```python
from build123d import *

# Parameters (mm, degrees)
F0_W     = 190
F0_H     = 20
F1_DEPTH = 4
F2_R     = 6
F3_DEPTH = 4.001
F4_R     = 9.99999


# Not quite as in the source:
# - a fillet or chamfer is up to 0.001 mm smaller than in the source, because OpenCascade refuses the exact size


with BuildPart() as f1:
    # F0 (on Top) → F1 (new body)
    with BuildSketch(Plane.XY):
        Rectangle(F0_W, F0_H)
    extrude(amount=F1_DEPTH)

    # F2 (on face) → F3 (cut, through all)
    with BuildSketch(Plane.XY.offset(4)):
        with Locations((-85, 0)):
            Circle(F2_R)
        with Locations((27, 0)):
            Circle(F2_R)
    extrude(amount=-F3_DEPTH, mode=Mode.SUBTRACT)

    # F4 (radius 10 in the source; OpenCascade refuses exactly that, so slightly less here)
    f4_edges = [f1.edges().sort_by_distance(p)[0] for p in [
        (-95, -10, 2),
        (-95, 10, 2),
        (95, 10, 2),
        (95, -10, 2),
    ]]
    fillet(f4_edges, radius=F4_R)


solid = f1.part
```
Part model, mm, in its own coordinate system. Round coordinates to 2 decimals unless told otherwise and drop trailing zeros. Loops run counter-clockwise (first coordinate to the right, second up) from the corner with the lowest first, then second, coordinate; pieces in that order, holes last. Notation, with made-up numbers: (89.5, 24.25) -> (136.5, 24.25) arc R20 cw to (136.5, 41.25) -> close; hole circle Ø3 at (12.5, -9). An arc over 180 degrees is marked (long way). Use a Markdown table: item, result.
1) Cut at A-A, the plane y = -2.75. List the corners of the cut face in (x, z), and give its area (3 significant figures).
The answers:
| item | result |
|---|---|
| outline | (-94.61, 0) -> (-90.33, 0) -> (-90.33, 4) -> (-94.61, 4) -> close; (-79.67, 0) -> (21.67, 0) -> (21.67, 4) -> (-79.67, 4) -> close; (32.33, 0) -> (94.61, 0) -> (94.61, 4) -> (32.33, 4) -> close |
| area | 672 mm2 |
2) Cut at C-C, the plane z = 0.85. State how many separate pieces and enclosed holes the cut face has, and give its area (3 significant figures).
The answers:
| item | result |
|---|---|
| separate pieces | 1 |
| enclosed holes | 2 |
| area | 3,490 mm2 |
3) Drop flat-ended pins along their axis: pin 1 Ø1 at (y, z) = (-7, 3) entering from -X; pin 2 Ø1.5 at (x, y) = (-66.5, 5.5) entering from -Z. Give the stop position or say it passes through.
The answers:
| item | result |
|---|---|
| pin 1 | stops at x = -92.6 |
| pin 2 | stops at z = 0 |
4) Cut at D-D, the plane x = -82.5. List the corners of the cut face in (y, z), and give its area (3 significant figures).
The answers:
| item | result |
|---|---|
| outline | (-10, 0) -> (-5.45, 0) -> (-5.45, 4) -> (-10, 4) -> close; (5.45, 0) -> (10, 0) -> (10, 4) -> (5.45, 4) -> close |
| area | 36.4 mm2 |
5) Cut at B-B, the plane x = 27. List the corners of the cut face in (y, z).
The answers:
| item | result |
|---|---|
| outline | (-10, 0) -> (-6, 0) -> (-6, 4) -> (-10, 4) -> close; (6, 0) -> (10, 0) -> (10, 4) -> (6, 4) -> close |
6) Pull direction Y, two halves, no side cores. Call faces 1 (the cylindrical face through (-91, 0, 2)), 2 (the flat face through (-1, 10, 2)), 3 (the flat face through (-1, -10, 2)): pulls with the +Y half, pulls with the -Y half, needs draft (parallel to the pull), parting line crosses it, or undercut.
The answers:
| item | result |
|---|---|
| face 1 | undercut |
| face 2 | pulls with the +Y half |
| face 3 | pulls with the -Y half |
7) Probe line 1 (X direction, y = 2, z = 3.7); line 2 (X direction, y = -2.25, z = 2.45); line 3 (Y direction, x = 27, z = 1.2). List the from-to ranges inside material, lowest first. Write a range as [from, to].
The answers:
| item | result |
|---|---|
| line 1 | x = [-94.8, -90.66], [-79.34, 21.34], [32.66, 94.8] |
| line 2 | x = [-94.74, -90.56], [-79.44, 21.44], [32.56, 94.74] |
| line 3 | y = [-10, -6], [6, 10] |
